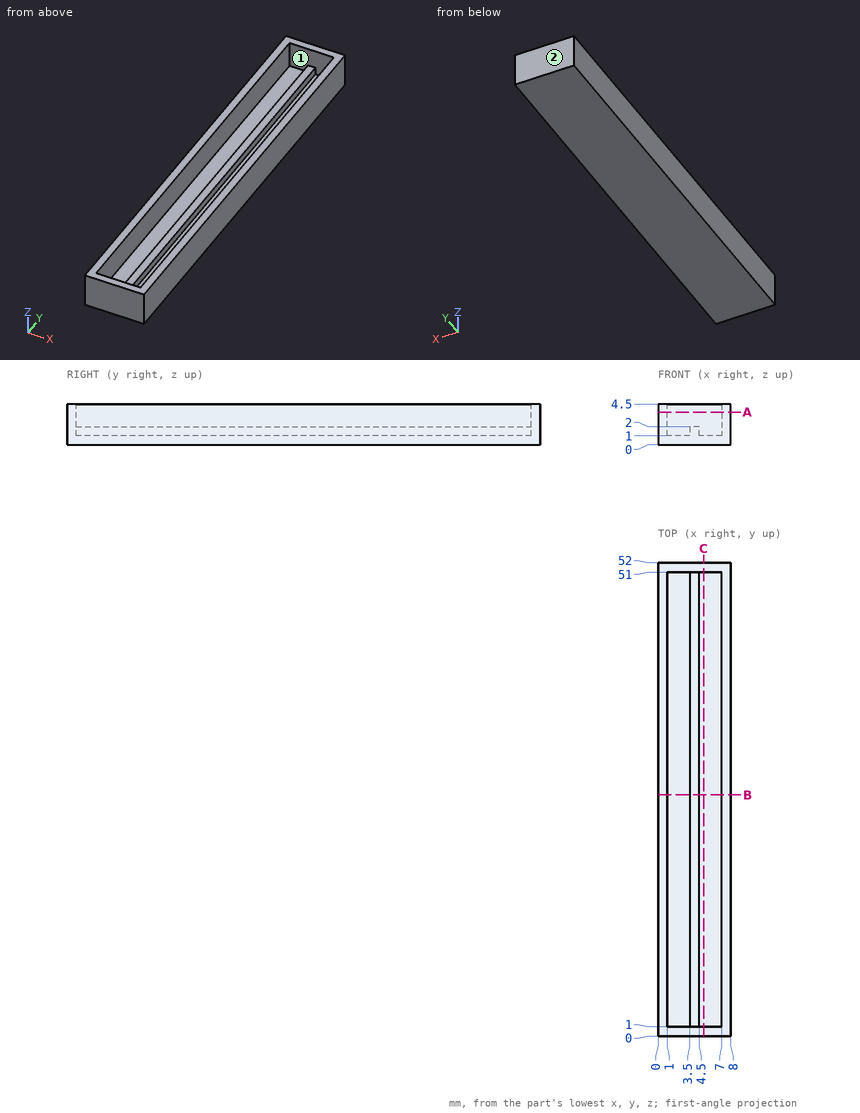
Check sheet for the drawn part. Datum: minimum x, y, z corner. Units: mm. A direction names the side the tool comes from. Give positions to 0.01 mm unless a question says otherwise; leave off trailing zeros. Write each loop counter-clockwise with the first axis right and the second up, starting at its lowest first coordinate (ties: lowest second). Pieces come first, ordered by that corner, then holes. Notation, with made-up numbers: (-36.5, -39.5) -> (-20.5, -39.5) arc R36 ccw to (-20.5, -4.5) -> close; hole circle Ø10 at (23, 78.5). An arc over 180 degrees is marked (long way). Use one line per item in the form item = value. Start each with the question number.
1. Go/stop test with flat-tipped pins: P1, Ø0.5, axis at x = 4, y = 17, coming from the +Z side; P2, Ø0.8, axis at x = 2.5, y = 37.5, coming from the +Z side. Record where each tip stops, or that it passes through.
2. Access from +Z, -Z, +X, -X, +Y, -Y to the whole of each face (thin tool, end or side, straight path). Record for the marked faces 1 and 2.
3. Section check B-B (y = 26.5). Record the cut outline in (x, z).
4. Thickness scan on line 1 along X through (y, z) = (10, 1.35); line 2 along X through (y, z) = (46, 3.6); line 3 along Y through (x, z) = (5.25, 3.3). Record the ranges inside material, lowest first. Write a range as from..to.
5. Section check A-A (z = 3.6). Record the cut outline in (x, y).
6. Section check C-C (x = 5). Record the cut outline in (y, z), and give its area (3 significant figures).
Conclusion:
q1.P1 = 2
q1.P2 = 1
q2.face_1 = +Z
q2.face_2 = +Z, -Z, +X, -X, +Y
q3.outline = (0, 0) -> (8, 0) -> (8, 4.5) -> (7, 4.5) -> (7, 1) -> (4.5, 1) -> (4.5, 2) -> (3.5, 2) -> (3.5, 1) -> (1, 1) -> (1, 4.5) -> (0, 4.5) -> close
q4.line_1 = 0..1, 3.5..4.5, 7..8
q4.line_2 = 0..1, 7..8
q4.line_3 = 0..1, 51..52
q5.outline = (0, 0) -> (8, 0) -> (8, 52) -> (0, 52) -> close; hole (1, 1) -> (7, 1) -> (7, 51) -> (1, 51) -> close
q6.outline = (0, 0) -> (52, 0) -> (52, 4.5) -> (51, 4.5) -> (51, 1) -> (1, 1) -> (1, 4.5) -> (0, 4.5) -> close
q6.area = 59.0 mm²
